Geometry check sheet. Reference: the model listing, model coordinates, mm. Coordinates: 2 decimals unless noted, no trailing zeros. Write each loop counter-clockwise with the first axis right and the second up, starting at its lowest first coordinate (ties: lowest second). Pieces come first, ordered by that corner, then holes. Notation, with made-up numbers: (-12, 51) -> (21, 51) arc R29 cw to (21, 80) -> close; hole circle Ø4 at (70.5, 19). An arc over 180 degrees is marked (long way). One line per question, with ' | ' between items.
```python
from build123d import *

# Parameters (mm, degrees)
SKETCH1_W           = 100
SKETCH1_H           = 40
BOSS_EXTRUDE2_DEPTH = 3.175


with BuildPart() as part:
    # Sketch1 → Boss-Extrude2 (new body)
    with BuildSketch(Plane(origin=(0, 0, 0), x_dir=(1, 0, 0), z_dir=(0, 1, 0))):
        with BuildLine():
            Line((-69.375, 37.5), (69.375, 37.5))
            ThreePointArc((69.375, 37.5), (76.446067812, 34.571067812), (79.375, 27.5))
            Line((79.375, 27.5), (82.55, 27.5))
            Line((82.55, 27.5), (82.55, 22.5))
            Line((82.55, 22.5), (85.725, 22.5))
            Line((85.725, 22.5), (85.725, 27.5))
            ThreePointArc((85.725, 27.5), (91.028300859, 25.303300859), (93.225, 20))
            Line((93.225, 20), (93.225, -20))
            ThreePointArc((93.225, -20), (91.028300859, -25.303300859), (85.725, -27.5))
            Line((85.725, -27.5), (85.725, -22.5))
            Line((85.725, -22.5), (82.55, -22.5))
            Line((82.55, -22.5), (82.55, -27.5))
            Line((82.55, -27.5), (79.375, -27.5))
            ThreePointArc((79.375, -27.5), (76.446067812, -34.571067812), (69.375, -37.5))
            Line((69.375, -37.5), (-69.375, -37.5))
            ThreePointArc((-69.375, -37.5), (-76.446067812, -34.571067812), (-79.375, -27.5))
            Line((-79.375, -27.5), (-82.55, -27.5))
            Line((-82.55, -27.5), (-82.55, -22.5))
            Line((-82.55, -22.5), (-85.725, -22.5))
            Line((-85.725, -22.5), (-85.725, -27.5))
            ThreePointArc((-85.725, -27.5), (-91.028300859, -25.303300859), (-93.225, -20))
            Line((-93.225, -20), (-93.225, 20))
            ThreePointArc((-93.225, 20), (-91.028300859, 25.303300859), (-85.725, 27.5))
            Line((-85.725, 27.5), (-85.725, 22.5))
            Line((-85.725, 22.5), (-82.55, 22.5))
            Line((-82.55, 22.5), (-82.55, 27.5))
            Line((-82.55, 27.5), (-79.375, 27.5))
            ThreePointArc((-79.375, 27.5), (-76.446067812, 34.571067812), (-69.375, 37.5))
        make_face()
        Rectangle(SKETCH1_W, SKETCH1_H, mode=Mode.SUBTRACT)
    extrude(amount=BOSS_EXTRUDE2_DEPTH)


solid = part.part
```
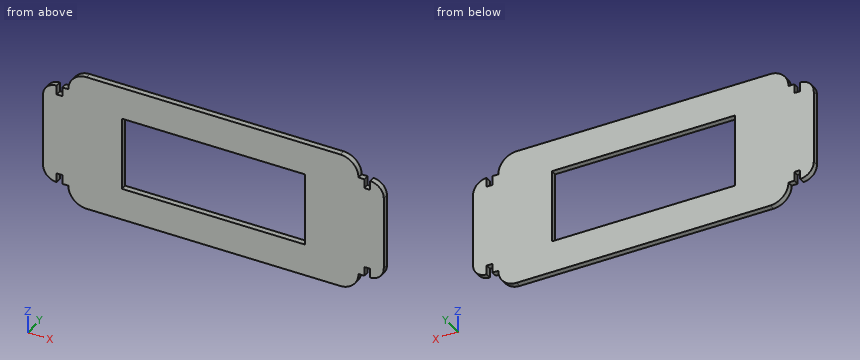
(1) Material ranges on line 1 (X direction, y = 1.3, z = 4) (3 decimals); line 2 (X direction, y = 1.75, z = -25) (3 decimals); line 3 (Z direction, x = 22.5, y = 0.7), recorded low to high.
Answers below:
line 1: x = -93.225 to -50, 50 to 93.225 | line 2: x = -91.315 to -85.725, -82.55 to 82.55, 85.725 to 91.315 | line 3: z = -37.5 to -20, 20 to 37.5
(2) Depth check by flat-ended pin: P1, Ø1.6, axis at y = 2, z = 24, coming from the -X side; P2, Ø1, axis at x = 80.5, y = 1.5, coming from the +Z side; P3, Ø1, axis at x = -83.5, y = 1.5, coming from the +Z side. Enter the tip coordinate at first touch or a pass-through.
Answers below:
P1: stops at x = -92.51 | P2: stops at z = 27.5 | P3: stops at z = 22.5
(3) Cross-section at C-C (x = 31.5). Record the cut outline in (y, z) (3 decimals).
Answers below:
outline: (0, -37.5) -> (3.175, -37.5) -> (3.175, -20) -> (0, -20) -> close; (0, 20) -> (3.175, 20) -> (3.175, 37.5) -> (0, 37.5) -> close
(4) Cross-section at D-D (z = 30). Record the cut outline in (x, y) (3 decimals).
Answers below:
outline: (-79.057, 0) -> (79.057, 0) -> (79.057, 3.175) -> (-79.057, 3.175) -> close
(5) Cross-section at A-A (z = 5.5). Record the cut outline in (x, y) (3 decimals).
Answers below:
outline: (-93.225, 0) -> (-50, 0) -> (-50, 3.175) -> (-93.225, 3.175) -> close; (50, 0) -> (93.225, 0) -> (93.225, 3.175) -> (50, 3.175) -> close
